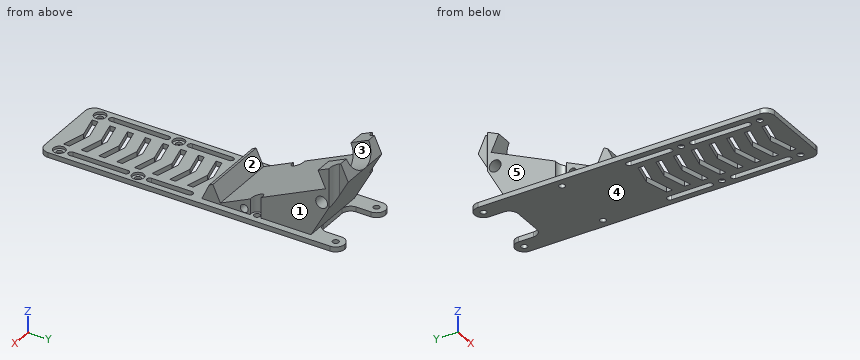
from build123d import *

# Parameters (mm, degrees)
F1_R          = 2
F1_R_2        = 3
F2_DEPTH      = 17.5
F2_DEPTH_BACK = 17.5
F3_R          = 9
F4_DEPTH      = 25
F0_R          = 1.55
F5_DEPTH      = 2.5
F6_R          = 3
F6_R_2        = 1.55
F6_R_3        = 2.9
F7_DEPTH      = 50
F9_DEPTH      = 25
F11_DEPTH     = 50
F12_DEPTH     = 1.25


with BuildPart() as f2:
    # F1 (on Right) → F2 (new body, two sides)
    with BuildSketch(Plane.YZ) as f2_sk:
        Polygon((8.5985827647, 10.6567700833), (12.4021471204, 2.5), (14.2147626945, 3.3452365235), (10.4111983388, 11.5020066068), align=None)
        Polygon((63.883357774, 36.4364840495), (67.6869221296, 28.2797139662), (76.75, 32.5058965836), (72.9464356443, 40.6626666669), align=None)
        Polygon((14.2147626945, 3.3452365235), (12.4021471204, 2.5), (60.25, 2.5), (76.75, 32.5058965836), (67.6869221296, 28.2797139662), align=None)
        with Locations((26.3704179861, 4.6)):
            Circle(F1_R, mode=Mode.SUBTRACT)
        with Locations((65.6910927649, 20.7287759353)):
            Circle(F1_R_2, mode=Mode.SUBTRACT)
        Polygon((8.5985827647, 2.5), (12.4021471204, 2.5), (8.5985827647, 10.6567700833), align=None)
        Polygon((8.5985827647, 2.5), (8.5985827647, 10.6567700833), (4.7950184091, 2.5), align=None)
    extrude(amount=F2_DEPTH)
    extrude(f2_sk.sketch, amount=-F2_DEPTH_BACK)

    # F3 (on face) → F4 (cut)
    with BuildSketch(Plane(origin=(0, 75.492455245, 35.2027100136), x_dir=(-1, 0, 0), z_dir=(0, 0.906307787, 0.4226182617))):
        with Locations((0, 6.0243956097)):
            Circle(F3_R)
    extrude(amount=-F4_DEPTH, mode=Mode.SUBTRACT)

    # F0 (on Top) → F5 (join)
    with BuildSketch(Plane.XY):
        with BuildLine():
            Line((21, -71.25), (21, 72.25))
            ThreePointArc((21, 72.25), (19.6819805153, 75.4319805153), (16.5, 76.75))
            ThreePointArc((16.5, 76.75), (13.3180194847, 75.4319805153), (12, 72.25))
            Line((12, 72.25), (12, 64.75))
            ThreePointArc((12, 64.75), (10.6819805153, 61.5680194847), (7.5, 60.25))
            Line((7.5, 60.25), (-7.5, 60.25))
            ThreePointArc((-7.5, 60.25), (-10.6819805153, 61.5680194847), (-12, 64.75))
            Line((-12, 64.75), (-12, 72.25))
            ThreePointArc((-12, 72.25), (-13.3180194847, 75.4319805153), (-16.5, 76.75))
            ThreePointArc((-16.5, 76.75), (-19.6819805153, 75.4319805153), (-21, 72.25))
            Line((-21, 72.25), (-21, -71.25))
            ThreePointArc((-21, -71.25), (-19.6819805153, -74.4319805153), (-16.5, -75.75))
            Line((-16.5, -75.75), (16.5, -75.75))
            ThreePointArc((16.5, -75.75), (19.6819805153, -74.4319805153), (21, -71.25))
        make_face()
        with Locations((-16.5, -68.25)):
            Circle(F0_R, mode=Mode.SUBTRACT)
        with BuildLine():
            ThreePointArc((-16.5, -32.75), (-15.4393398282, -33.1893398282), (-15, -34.25))
            Line((-15, -34.25), (-15, -62.25))
            ThreePointArc((-15, -62.25), (-15.4393398282, -63.3106601718), (-16.5, -63.75))
            ThreePointArc((-16.5, -63.75), (-17.5606601718, -63.3106601718), (-18, -62.25))
            Line((-18, -62.25), (-18, -34.25))
            ThreePointArc((-18, -34.25), (-17.5606601718, -33.1893398282), (-16.5, -32.75))
        make_face(mode=Mode.SUBTRACT)
        with Locations((-16.5, -28.25)):
            Circle(F0_R, mode=Mode.SUBTRACT)
        with BuildLine():
            ThreePointArc((-16.5, -0.25), (-15.4393398282, -0.6893398282), (-15, -1.75))
            Line((-15, -1.75), (-15, -22.25))
            ThreePointArc((-15, -22.25), (-15.4393398282, -23.3106601718), (-16.5, -23.75))
            ThreePointArc((-16.5, -23.75), (-17.5606601718, -23.3106601718), (-18, -22.25))
            Line((-18, -22.25), (-18, -1.75))
            ThreePointArc((-18, -1.75), (-17.5606601718, -0.6893398282), (-16.5, -0.25))
        make_face(mode=Mode.SUBTRACT)
        with Locations((16.5, -68.25)):
            Circle(F0_R, mode=Mode.SUBTRACT)
        with BuildLine():
            Line((15, -62.25), (15, -34.25))
            ThreePointArc((15, -34.25), (15.4393398282, -33.1893398282), (16.5, -32.75))
            ThreePointArc((16.5, -32.75), (17.5606601718, -33.1893398282), (18, -34.25))
            Line((18, -34.25), (18, -62.25))
            ThreePointArc((18, -62.25), (17.5606601718, -63.3106601718), (16.5, -63.75))
            ThreePointArc((16.5, -63.75), (15.4393398282, -63.3106601718), (15, -62.25))
        make_face(mode=Mode.SUBTRACT)
        with Locations((16.5, -28.25)):
            Circle(F0_R, mode=Mode.SUBTRACT)
        with BuildLine():
            Line((15, -22.25), (15, -1.75))
            ThreePointArc((15, -1.75), (15.4393398282, -0.6893398282), (16.5, -0.25))
            ThreePointArc((16.5, -0.25), (17.5606601718, -0.6893398282), (18, -1.75))
            Line((18, -1.75), (18, -22.25))
            ThreePointArc((18, -22.25), (17.5606601718, -23.3106601718), (16.5, -23.75))
            ThreePointArc((16.5, -23.75), (15.4393398282, -23.3106601718), (15, -22.25))
        make_face(mode=Mode.SUBTRACT)
        with Locations((-16.5, 32.25)):
            Circle(F0_R, mode=Mode.SUBTRACT)
        with Locations((-16.5, 72.25)):
            Circle(F0_R, mode=Mode.SUBTRACT)
        with Locations((16.5, 32.25)):
            Circle(F0_R, mode=Mode.SUBTRACT)
        with Locations((16.5, 72.25)):
            Circle(F0_R, mode=Mode.SUBTRACT)
    extrude(amount=F5_DEPTH)

    # F6 (on face) → F7 (cut)
    with BuildSketch(Plane.XY.offset(2.5)):
        with Locations((-16.5, -28.25)):
            Circle(F6_R)
        with Locations((-16.5, -28.25)):
            Circle(F6_R_2, mode=Mode.SUBTRACT)
        with Locations((16.5, -28.25)):
            Circle(F6_R)
        with Locations((16.5, -28.25)):
            Circle(F6_R_2, mode=Mode.SUBTRACT)
        with Locations((-16.5, -68.25)):
            Circle(F6_R)
        with Locations((-16.5, -68.25)):
            Circle(F6_R_2, mode=Mode.SUBTRACT)
        with Locations((16.5, -68.25)):
            Circle(F6_R)
        with Locations((16.5, -68.25)):
            Circle(F6_R_2, mode=Mode.SUBTRACT)
        with Locations((16.5, 72.25)):
            Circle(F6_R_3)
        with Locations((16.5, 72.25)):
            Circle(F6_R_2, mode=Mode.SUBTRACT)
        with Locations((-16.5, 72.25)):
            Circle(F6_R_3)
        with Locations((-16.5, 72.25)):
            Circle(F6_R_2, mode=Mode.SUBTRACT)
        with BuildLine():
            ThreePointArc((-17.5, 29.5278684822), (-14.8401807327, 29.8719756099), (-13.6, 32.25))
            ThreePointArc((-13.6, 32.25), (-14.8401807327, 34.6280243901), (-17.5, 34.9721315178))
            Line((-17.5, 34.9721315178), (-17.5, 33.4342719282))
            ThreePointArc((-17.5, 33.4342719282), (-18.05, 32.25), (-17.5, 31.0657280718))
            Line((-17.5, 31.0657280718), (-17.5, 29.5278684822))
        make_face()
        with BuildLine():
            ThreePointArc((17.5, 34.9721315178), (13.6, 32.25), (17.5, 29.5278684822))
            Line((17.5, 29.5278684822), (17.5, 31.0657280718))
            ThreePointArc((17.5, 31.0657280718), (17.905791592, 31.5971217571), (18.05, 32.25))
            ThreePointArc((18.05, 32.25), (17.905791592, 32.9028782429), (17.5, 33.4342719282))
            Line((17.5, 33.4342719282), (17.5, 34.9721315178))
        make_face()
        with Locations((16.5, -28.25)):
            Circle(F6_R_2)
        with Locations((-16.5, -28.25)):
            Circle(F6_R_2)
        with Locations((-16.5, -68.25)):
            Circle(F6_R_2)
        with Locations((16.5, -68.25)):
            Circle(F6_R_2)
        with Locations((16.5, 72.25)):
            Circle(F6_R_2)
        with Locations((-16.5, 72.25)):
            Circle(F6_R_2)
        with BuildLine():
            Line((-17.5, 33.4342719282), (-17.5, 34.9721315178))
            ThreePointArc((-17.5, 34.9721315178), (-19.4, 32.25), (-17.5, 29.5278684822))
            Line((-17.5, 29.5278684822), (-17.5, 31.0657280718))
            ThreePointArc((-17.5, 31.0657280718), (-18.05, 32.25), (-17.5, 33.4342719282))
        make_face()
        with BuildLine():
            Line((17.5, 31.0657280718), (17.5, 29.5278684822))
            ThreePointArc((17.5, 29.5278684822), (18.8780243901, 30.5901807327), (19.4, 32.25))
            ThreePointArc((19.4, 32.25), (18.8780243901, 33.9098192673), (17.5, 34.9721315178))
            Line((17.5, 34.9721315178), (17.5, 33.4342719282))
            ThreePointArc((17.5, 33.4342719282), (17.905791592, 32.9028782429), (18.05, 32.25))
            ThreePointArc((18.05, 32.25), (17.905791592, 31.5971217571), (17.5, 31.0657280718))
        make_face()
    extrude(amount=F7_DEPTH, mode=Mode.SUBTRACT)

    # F8 (on face) → F9 (cut)
    with BuildSketch(Plane.XY.offset(2.5)):
        Polygon((11.6, -3.25), (0, -0.25), (-11.6, -3.25), (-11.6, -6.25), (0, -3.25), (11.6, -6.25), align=None)
        Polygon((0, -9.25), (-11.6, -12.25), (-11.6, -15.25), (0, -12.25), (11.6, -15.25), (11.6, -12.25), align=None)
        Polygon((0, -18.25), (-11.6, -21.25), (-11.6, -24.25), (0, -21.25), (11.6, -24.25), (11.6, -21.25), align=None)
        Polygon((0, -27.25), (-11.6, -30.25), (-11.6, -33.25), (0, -30.25), (11.6, -33.25), (11.6, -30.25), align=None)
        Polygon((0, -36.25), (-11.6, -39.25), (-11.6, -42.25), (0, -39.25), (11.6, -42.25), (11.6, -39.25), align=None)
        Polygon((0, -45.25), (-11.6, -48.25), (-11.6, -51.25), (0, -48.25), (11.6, -51.25), (11.6, -48.25), align=None)
        Polygon((0, -54.25), (-11.6, -57.25), (-11.6, -60.25), (0, -57.25), (11.6, -60.25), (11.6, -57.25), align=None)
        Polygon((0, -63.25), (-11.6, -66.25), (-11.6, -69.25), (0, -66.25), (11.6, -69.25), (11.6, -66.25), align=None)
    extrude(amount=-F9_DEPTH, mode=Mode.SUBTRACT)

    # F10 (on face) → F11 (cut)
    with BuildSketch(Plane.XY.offset(2.5)):
        with BuildLine():
            ThreePointArc((14.95, 72.25), (15.6128552192, 73.5210130361), (17.0344827586, 73.7049323629))
            Line((17.0344827586, 73.7049323629), (17.5, 74.9721315178))
            Line((17.5, 74.9721315178), (17.5, 76.6374821937))
            ThreePointArc((17.5, 76.6374821937), (17.0031551095, 76.7217820761), (16.5, 76.75))
            ThreePointArc((16.5, 76.75), (14.9563331772, 76.4769483958), (13.6, 75.6909301068))
            Line((13.6, 75.6909301068), (13.6, 72.25))
            Line((13.6, 72.25), (14.95, 72.25))
        make_face()
        with BuildLine():
            Line((13.6, 76.75), (13.6, 75.6909301068))
            ThreePointArc((13.6, 75.6909301068), (14.9563331772, 76.4769483958), (16.5, 76.75))
            Line((16.5, 76.75), (13.6, 76.75))
        make_face()
        with BuildLine():
            Line((-13.6, 76.75), (-16.5, 76.75))
            ThreePointArc((-16.5, 76.75), (-14.9563331772, 76.4769483958), (-13.6, 75.6909301068))
            Line((-13.6, 75.6909301068), (-13.6, 76.75))
        make_face()
        with BuildLine():
            ThreePointArc((-16.5, 76.75), (-17.0031551095, 76.7217820761), (-17.5, 76.6374821937))
            Line((-17.5, 76.6374821937), (-17.5, 74.9721315178))
            Line((-17.5, 74.9721315178), (-17.0344827586, 73.7049323629))
            ThreePointArc((-17.0344827586, 73.7049323629), (-15.6128552192, 73.5210130361), (-14.95, 72.25))
            Line((-14.95, 72.25), (-13.6, 72.25))
            Line((-13.6, 72.25), (-13.6, 75.6909301068))
            ThreePointArc((-13.6, 75.6909301068), (-14.9563331772, 76.4769483958), (-16.5, 76.75))
        make_face()
        with BuildLine():
            Line((-17.5, 76.75), (-17.5, 76.6374821937))
            ThreePointArc((-17.5, 76.6374821937), (-17.0031551095, 76.7217820761), (-16.5, 76.75))
            Line((-16.5, 76.75), (-17.5, 76.75))
        make_face()
        with BuildLine():
            ThreePointArc((16.5, 76.75), (17.0031551095, 76.7217820761), (17.5, 76.6374821937))
            Line((17.5, 76.6374821937), (17.5, 76.75))
            Line((17.5, 76.75), (16.5, 76.75))
        make_face()
    extrude(amount=F11_DEPTH, mode=Mode.SUBTRACT)

    # F6 (on face) → F12 (cut)
    with BuildSketch(Plane.XY.offset(2.5)):
        with Locations((-16.5, -28.25)):
            Circle(F6_R)
        with Locations((-16.5, -28.25)):
            Circle(F6_R_2, mode=Mode.SUBTRACT)
        with Locations((16.5, -28.25)):
            Circle(F6_R)
        with Locations((16.5, -28.25)):
            Circle(F6_R_2, mode=Mode.SUBTRACT)
        with Locations((16.5, -68.25)):
            Circle(F6_R)
        with Locations((16.5, -68.25)):
            Circle(F6_R_2, mode=Mode.SUBTRACT)
        with Locations((-16.5, -68.25)):
            Circle(F6_R)
        with Locations((-16.5, -68.25)):
            Circle(F6_R_2, mode=Mode.SUBTRACT)
    extrude(amount=-F12_DEPTH, mode=Mode.SUBTRACT)


solid = f2.part
Geometry: final body of the model. Coordinates: model frame, mm. Face numbers are marked on the shaded views. A direction names the side the tool comes from. Round coordinates to 2 decimals unless told otherwise and drop trailing zeros. Loops run counter-clockwise (first coordinate to the right, second up) from the corner with the lowest first, then second, coordinate; pieces in that order, holes last.
Q1. Pull-direction query (Y, two-part tool) for the marked faces 1, 2 and 3; classes: released by +Y, released by -Y, zero draft, split by the parting line, or undercut.
Q2. Pin query (flat end, axial travel): P1, Ø5, axis at x = 6.5, z = 11, coming from the -Y side; P2, Ø10, axis at y = 13.5, z = 9, coming from the +X side; P3, Ø1.3, axis at y = 74, z = 34, coming from the +X side. Return the tip coordinate at first contact, or that it passes through.
Q3. Section B-B on x = 3.5. State how many separate pieces and enclosed holes the cut face has, plus the area to 3 significant figures.
Q4. Material intervals for L1, parallel to Z at x = -7, y = 0.5; L2, parallel to Y at x = -16.5, z = 7.5; L3, parallel to X at y = 32, z = 7, sorted ascending.
Q5. Section C-C on y = 41. Return loops of the section in (x, z).
Q6. Section A-A on z = 8. Return loops of the section in (x, y).
Q7. Access query for the marked faces 4 and 5. Directions: +Z, -Z, +X, -X, +Y, -Y. A direction counts if a zero-diameter tool reaches every point of the face in a straight line with its end or side. Return the directions, or none.
Evaluation:
1. face 1: zero draft
1. face 2: undercut
1. face 3: released by -Y
2. P1: stops at y = 7.59
2. P2: stops at x = 17.5
2. P3: stops at x = 13.6
3. separate pieces: 9
3. enclosed holes: 2
3. area: 1,010 mm2
4. L1: z = 0 to 2.5
4. L2: y = 7.13 to 12.28, 23.12 to 29.35, 35.15 to 63
4. L3: x = -13.61 to 13.61
5. outline: (-21, 0) - (21, 0) - (21, 2.5) - (17.5, 2.5) - (17.5, 15.84) - (-17.5, 15.84) - (-17.5, 2.5) - (-21, 2.5) - close
6. outline: (-17.5, 7.36) - (17.5, 7.36) - (17.5, 12.04) - (-17.5, 12.04) - close; (-17.5, 24.2) - (17.5, 24.2) - (17.5, 29.53) arc R2.9 cw (long way) to (17.5, 34.97) - (17.5, 63.27) - (-17.5, 63.27) - (-17.5, 34.97) arc R2.9 cw (long way) to (-17.5, 29.53) - close
7. face 4: -Z, +X, -X, +Y, -Y
7. face 5: +Z, -X, +Y, -Y
